Source: CAD feature listing. Evaluate the final solid. Frame: model axes, mm. Face numbers are marked on the shaded views. A direction names the side the tool comes from. Give positions to 0.01 mm unless a question says otherwise; leave off trailing zeros. Order: outer loops, then holes, each group sorted by start corner. A loop starts at its lowest first (then second) coordinate and runs counter-clockwise, first axis right, second up. Notation, with made-up numbers: M -10,8.5 L 45,8.5 A11 cw 45,23.5 Z; hole C 0,20.5 d8. An arc over 180 degrees is marked long. Use CSV: the item, a comma, the result in double quotes. Start each with the question number.
1. Section query B-B, the plane y = -14. Return the cut outline in (x, z), plus the area to 3 significant figures.
2. Line query: line 1 along Y through (x, z) = (51.86, 0.8); line 2 along X through (y, z) = (-21.5, 7.25); line 3 along X through (y, z) = (-5, 7). Output: solid intervals per line, ascending. Write a range as [from, to].
3. Mould query, pull axis X, two halves, no side actions, for the marked faces 1, 2, 3 and 4. Classes: released by +X, released by -X, zero draft, split by the parting line, or undercut.
4. Section query A-A, the plane x = -24.5. Return the cut outline in (y, z).
5. Section query C-C, the plane x = 3. Return the cut outline in (y, z).
6. Pin query (flat end, axial travel): P1, Ø1.8, axis at x = -59.5, y = -8, coming from the -Z side; P2, Ø3.5, axis at x = -53, y = -21.5, coming from the -Z side; P3, Ø6, axis at x = -7.5, z = 7, coming from the -Y side. Return the tip coordinate at first contact, or that it passes through.
7. Reachability of the marked faces 5 and 6 from +Z, -Z, +X, -X, +Y, -Y: full face, straight path, thin tool, end or side. Return the list, or none.
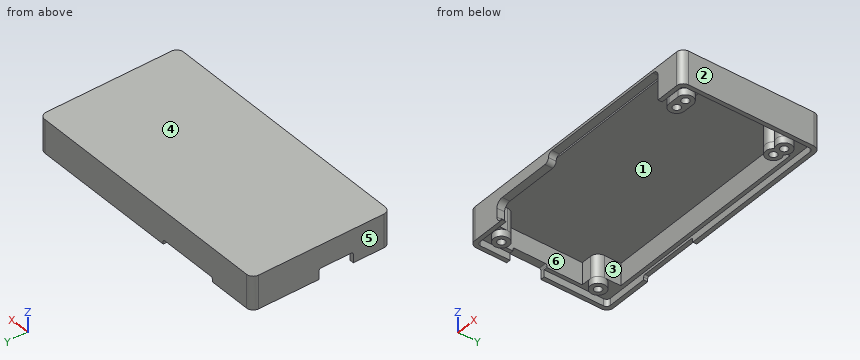
from build123d import *

# Parameters (mm, degrees)
PAD006_DEPTH    = 3.2
SKETCH009_W     = 114.2
SKETCH009_H     = 56
PAD007_DEPTH    = 10
PAD008_DEPTH    = 2
POCKET002_DEPTH = 5
POCKET003_DEPTH = 5
POCKET004_DEPTH = 3.5
SKETCH014_R     = 1.5
PAD009_DEPTH    = 10
SKETCH015_R     = 3.5
SKETCH015_R_2   = 1.7
PAD010_DEPTH    = 3.1


with BuildPart() as part:
    # Sketch008 → Pad006 (new body)
    with BuildSketch(Plane.XY):
        with BuildLine():
            Line((56.86, 33.5), (-58.34, 33.5))
            ThreePointArc((-58.34, 33.5), (-60.46132, 32.62132), (-61.34, 30.5))
            Line((-61.34, 30.5), (-61.34, -26.5))
            ThreePointArc((-61.34, -26.5), (-60.46132, -28.62132), (-58.34, -29.5))
            Line((-58.34, -29.5), (56.86, -29.5))
            ThreePointArc((56.86, -29.5), (58.98132, -28.62132), (59.86, -26.5))
            Line((59.86, -26.5), (59.86, 30.5))
            ThreePointArc((59.86, 30.5), (58.98132, 32.62132), (56.86, 33.5))
        make_face()
        with BuildLine():
            Line((56.26, 31.65), (-57.74, 31.65))
            ThreePointArc((-57.74, 31.65), (-58.977437, 31.137437), (-59.49, 29.9))
            Line((-59.49, 29.9), (-59.49, -25.9))
            ThreePointArc((-59.49, -25.9), (-58.977437, -27.137437), (-57.74, -27.65))
            Line((-57.74, -27.65), (56.26, -27.65))
            ThreePointArc((56.26, -27.65), (57.497437, -27.137437), (58.01, -25.9))
            Line((58.01, -25.9), (58.01, 29.9))
            ThreePointArc((58.01, 29.9), (57.497437, 31.137437), (56.26, 31.65))
        make_face(mode=Mode.SUBTRACT)
    extrude(amount=PAD006_DEPTH)

    # Sketch009 (on Face18 of Pad006) → Pad007 (join)
    with BuildSketch(Plane.XY.offset(3.2)):
        with BuildLine():
            Line((-61.34, 30.5), (-61.34, -26.5))
            ThreePointArc((-61.34, -26.5), (-60.46132, -28.62132), (-58.34, -29.5))
            Line((-58.34, -29.5), (56.86, -29.5))
            ThreePointArc((56.86, -29.5), (58.98132, -28.62132), (59.86, -26.5))
            Line((59.86, -26.5), (59.86, 30.5))
            ThreePointArc((59.86, 30.5), (58.98132, 32.62132), (56.86, 33.5))
            Line((56.86, 33.5), (-58.34, 33.5))
            ThreePointArc((-58.34, 33.5), (-60.46132, 32.62132), (-61.34, 30.5))
        make_face()
        with Locations((-0.74, 2)):
            Rectangle(SKETCH009_W, SKETCH009_H, mode=Mode.SUBTRACT)
    extrude(amount=PAD007_DEPTH)

    # Sketch010 (on Face12 of Pad007) → Pad008 (join)
    with BuildSketch(Plane.XY.offset(13.2)):
        with BuildLine():
            Line((-61.34, 30.5), (-61.34, -26.5))
            ThreePointArc((-61.34, -26.5), (-60.46132, -28.62132), (-58.34, -29.5))
            Line((-58.34, -29.5), (56.86, -29.5))
            ThreePointArc((56.86, -29.5), (58.98132, -28.62132), (59.86, -26.5))
            Line((59.86, -26.5), (59.86, 30.5))
            ThreePointArc((59.86, 30.5), (58.98132, 32.62132), (56.86, 33.5))
            Line((56.86, 33.5), (-58.34, 33.5))
            ThreePointArc((-58.34, 33.5), (-60.46132, 32.62132), (-61.34, 30.5))
        make_face()
    extrude(amount=PAD008_DEPTH)

    # Sketch011 (on Face18 of Pad008) → Pocket002 (cut)
    with BuildSketch(Plane(origin=(-61.34, 0, 0), x_dir=(0, -1, 0), z_dir=(-1, 0, 0))):
        with BuildLine():
            Line((-2.9, 0), (12.6, 0))
            Line((12.6, 0), (12.6, 4))
            ThreePointArc((12.6, 4), (12.38033, 4.53033), (11.85, 4.75))
            Line((11.85, 4.75), (-2.15, 4.75))
            ThreePointArc((-2.15, 4.75), (-2.68033, 4.53033), (-2.9, 4))
            Line((-2.9, 4), (-2.9, 0))
        make_face()
    extrude(amount=-POCKET002_DEPTH, mode=Mode.SUBTRACT)

    # Sketch012 (on Face20 of Pocket002) → Pocket003 (cut)
    with BuildSketch(Plane(origin=(0, 33.5, 0), x_dir=(-1, 0, 0), z_dir=(0, 1, 0))):
        with BuildLine():
            Line((10.74, 0), (38.74, 0))
            Line((38.74, 0), (38.74, 1.25))
            ThreePointArc((38.74, 1.25), (38.52033, 1.78033), (37.99, 2))
            Line((37.99, 2), (11.49, 2))
            ThreePointArc((11.49, 2), (10.95967, 1.78033), (10.74, 1.25))
            Line((10.74, 1.25), (10.74, 0))
        make_face()
    extrude(amount=-POCKET003_DEPTH, mode=Mode.SUBTRACT)

    # Sketch013 (on Face4 of Pocket003) → Pocket004 (cut)
    with BuildSketch(Plane.XZ.offset(29.5)):
        with BuildLine():
            ThreePointArc((-45.74, 3), (-44.86132, 0.87868), (-42.74, 0))
            Line((-16.34, 0), (-42.74, 0))
            ThreePointArc((-16.34, 0), (-15.754214, -1.414214), (-14.34, -2))
            Line((25.66, -2), (-14.34, -2))
            ThreePointArc((25.66, -2), (27.074214, -1.414214), (27.66, 0))
            Line((27.66, 0), (46.26, 0))
            Line((46.26, 0), (46.26, 3))
            Line((46.26, 11), (46.26, 3))
            ThreePointArc((46.26, 11), (45.38132, 13.12132), (43.26, 14))
            Line((43.26, 14), (-14.34, 14))
            ThreePointArc((-14.34, 14), (-15.754214, 13.414214), (-16.34, 12))
            ThreePointArc((-18.34, 10), (-16.925786, 10.585786), (-16.34, 12))
            Line((-42.74, 10), (-18.34, 10))
            ThreePointArc((-42.74, 10), (-44.86132, 9.12132), (-45.74, 7))
            Line((-45.74, 3), (-45.74, 7))
        make_face()
    extrude(amount=-POCKET004_DEPTH, mode=Mode.SUBTRACT)

    # Sketch014 (on Face43 of Pocket004) → Pad009 (join)
    with BuildSketch(Plane(origin=(0, 0, 13.2), x_dir=(1, 0, 0), z_dir=(0, 0, -1))):
        with BuildLine():
            ThreePointArc((-49.74, -22.5), (-50.765126, -20.025126), (-53.24, -19))
            Line((-57.84, -19), (-53.24, -19))
            Line((-57.84, -30), (-57.84, -19))
            Line((-57.84, -30), (-49.74, -30))
            Line((-49.74, -30), (-49.74, -22.5))
        make_face()
        with Locations((-53.24, -22.5)):
            Circle(SKETCH014_R, mode=Mode.SUBTRACT)
        with BuildLine():
            Line((-57.84, 26), (-57.84, 18))
            Line((-57.84, 18), (-53.24, 18))
            ThreePointArc((-53.24, 18), (-50.765126, 19.025126), (-49.74, 21.5))
            Line((-49.74, 21.5), (-49.74, 26))
            Line((-49.74, 26), (-57.84, 26))
        make_face()
        with Locations((-53.24, 21.5)):
            Circle(SKETCH014_R, mode=Mode.SUBTRACT)
        with BuildLine():
            Line((56.36, 26), (46.86, 26))
            Line((46.86, 25), (46.86, 26))
            ThreePointArc((46.86, 25), (43.36, 21.5), (46.86, 18))
            Line((46.86, 18), (56.36, 18))
            Line((56.36, 18), (56.36, 26))
        make_face()
        with Locations((46.86, 21.5)):
            Circle(SKETCH014_R, mode=Mode.SUBTRACT)
        with Locations((51.86, 21.5)):
            Circle(SKETCH014_R, mode=Mode.SUBTRACT)
        with BuildLine():
            Line((56.36, -30), (56.36, -23.4))
            Line((56.36, -23.4), (55.36, -23.4))
            ThreePointArc((55.36, -23.4), (53.440019, -20.276934), (49.786549, -20.580284))
            ThreePointArc((49.786549, -20.580284), (43.780308, -20.837022), (46.86, -26))
            Line((46.86, -26), (46.86, -30))
            Line((46.86, -30), (56.36, -30))
        make_face()
        with Locations((46.86, -22.5)):
            Circle(SKETCH014_R, mode=Mode.SUBTRACT)
        with Locations((51.86, -23.4)):
            Circle(SKETCH014_R, mode=Mode.SUBTRACT)
    extrude(amount=PAD009_DEPTH)

    # Sketch015 (on Face62 of Pad009) → Pad010 (join)
    with BuildSketch(Plane(origin=(0, 0, 3.2), x_dir=(1, 0, 0), z_dir=(0, 0, -1))):
        with Locations((-53.24, -22.5)):
            Circle(SKETCH015_R)
        with Locations((-53.24, -22.5)):
            Circle(SKETCH015_R_2, mode=Mode.SUBTRACT)
        with Locations((-53.24, 21.5)):
            Circle(SKETCH015_R)
        with Locations((-53.24, 21.5)):
            Circle(SKETCH015_R_2, mode=Mode.SUBTRACT)
        with BuildLine():
            ThreePointArc((46.86, 25), (43.36, 21.5), (46.86, 18))
            Line((46.86, 18), (51.86, 18))
            ThreePointArc((51.86, 18), (55.36, 21.5), (51.86, 25))
            Line((46.86, 25), (51.86, 25))
        make_face()
        with Locations((46.86, 21.5)):
            Circle(SKETCH015_R_2, mode=Mode.SUBTRACT)
        with Locations((51.86, 21.5)):
            Circle(SKETCH015_R_2, mode=Mode.SUBTRACT)
        with BuildLine():
            ThreePointArc((49.786549, -20.580284), (43.415358, -21.879965), (48.933451, -25.319716))
            ThreePointArc((48.933451, -25.319716), (55.304642, -24.020035), (49.786549, -20.580284))
        make_face()
        with Locations((51.86, -23.4)):
            Circle(SKETCH015_R_2, mode=Mode.SUBTRACT)
        with Locations((46.86, -22.5)):
            Circle(SKETCH015_R_2, mode=Mode.SUBTRACT)
    extrude(amount=PAD010_DEPTH)


solid = part.part
Result set:
1,outline,"M -61.34,0 L -59.49,0 L -59.49,3.2 L -57.84,3.2 L -57.84,13.2 L 56.36,13.2 L 56.36,3.2 L 58.01,3.2 L 58.01,0 L 59.86,0 L 59.86,15.2 L -61.34,15.2 Z"
1,area,"324 mm2"
2,line 1,"[-29.5, -27.65], [-25, -23.2], [-19.8, -18], [19.9, 21.7], [25.1, 26.9], [31.65, 33.5]"
2,line 2,"[-61.34, -54.74], [-51.74, -49.74], [43.36, 45.36], [48.36, 50.36], [53.36, 59.86]"
2,line 3,"[-61.34, -57.84], [56.36, 59.86]"
3,face 1,"undercut"
3,face 2,"released by +X"
3,face 3,"undercut"
3,face 4,"zero draft"
4,outline,"M -29.5,10 L -26,10 L -26,13.2 L 30,13.2 L 30,3.2 L 31.65,3.2 L 31.65,2 L 33.5,2 L 33.5,15.2 L -29.5,15.2 Z"
5,outline,"M -29.5,14 L -26,14 L -26,13.2 L 30,13.2 L 30,3.2 L 31.65,3.2 L 31.65,0 L 33.5,0 L 33.5,15.2 L -29.5,15.2 Z"
6,P1,"z = 4.75"
6,P2,"z = 0.1"
6,P3,"y = 30"
7,face 5,"+Z, -Z, -X, +Y, -Y"
7,face 6,"-Z"
